Autodesk Inventor part; units mm, degrees
ref_plane "YZ Plane" through (0, 0, 0) normal (1, 0, 0) x (0, 1, 0)
ref_plane "XZ Plane" through (0, 0, 0) normal (0, 1, 0) x (-1, 0, 0)
ref_plane "XY Plane" through (0, 0, 0) normal (0, 0, 1) x (1, 0, 0)
sketch "Sketch1" plane through (0, 0, 0) normal (0, 0, 1) x (1, 0, 0)
  arc A0 (58.1571, 20) -> (-58.1571, 20) centre (0, 0) ccw
  line L0 (-90, 0) -> (90, 0) construction
  line L1 (-90, 20) -> (90, 20)
  line L2 (-90, 23) -> (90, 23)
  line L3 (-90, 20) -> (-90, 23)
  line L4 (90, 20) -> (90, 23)
  arc A1 (61.3209, 20) -> (-61.3209, 20) centre (0, 0) ccw
  point P0 (60.2599, 23)
  point P1 (-60.2599, 23)
  dimension "d8" = 123
  dimension "d12" = 90
  dimension "d13" = 90
  dimension "d14" = 0
  dimension "d15" = 20
  dimension "d16" = 3
  dimension "d17" = 129
  dimension "d18" = 180
  dimension "d19" = 90
extrude "Extrusion2" add sketch "Sketch1" against normal blind 20 contours A0 L2 A1 L1 | A0 L2 A1 | L1 A1 L2 A0 | A1 L2 L4 L1 | L1 L3 L2 A1
sketch "Sketch2" plane through (60.2599, 23, 0) normal (0, 1, 0) x (1, 0, 0)
  circle A0 centre (14, 10) radius 5
  line L0 (29.7401, 0) -> (0, 0)
  point P0 (-60.2599, 0)
  dimension "d22" = 10
  dimension "d23" = 10
  dimension "d24" = 14
hole "Hole1" at (74.2599, 23, -10) direction (0, -1, 0) diameter 10 end through all
ref_plane "Work Plane1" through (0, 20, 0) normal (1, 0, 0) x (0, 0, -1)
thread "Thread1"
mirror "Mirror1" about plane through (0, 20, 0) normal (1, 0, 0) of "Hole1"
properties part number "Holder"
Read the model definition and answer for the solid it produces. Units are mm, in the model's axes. A direction names the side the tool comes from. Coordinates: 2 decimals unless noted, no trailing zeros. Write each loop counter-clockwise with the first axis right and the second up, starting at its lowest first coordinate (ties: lowest second). Pieces come first, ordered by that corner, then holes. Notation, with made-up numbers: M 23,83.25 L 46,83.25 A30 ccw 46,106.25 Z; hole C 16,-0.5 d11. An arc over 180 degrees is marked long. Use a Markdown table: item, result.
Q1. The part is cut by section A-A, the plane z = -10. Write down the section's boundary in (x, y), then the cut area to 3 significant figures.
Answer block:
| item | result |
|---|---|
| outline | M -90,20 L -79.26,20 L -79.26,23 L -90,23 Z; M -69.26,20 L -58.16,20 A61.5 cw 58.16,20 L 69.26,20 L 69.26,23 L 60.26,23 A64.5 ccw -60.26,23 L -69.26,23 Z; M 79.26,20 L 90,20 L 90,23 L 79.26,23 Z |
| area | 587 mm2 |
Q2. Determine the mould class of faces 4 (the face through (0, 62, 0)), 5 (the face through (1.07, 61.49, -9.86)), 6 (the face through (-90, 21, -10)) for opening direction X: released by +X, released by -X, zero draft, split by the parting line, or undercut.
Answer block:
| item | result |
|---|---|
| face 4 | zero draft |
| face 5 | undercut |
| face 6 | released by -X |
Q3. The part is cut by section B-B, the plane y = 33. Write down the section's boundary in (x, z), then the cut area to 3 significant figures.
Answer block:
| item | result |
|---|---|
| outline | M -55.42,-20 L -51.9,-20 L -51.9,0 L -55.42,0 Z; M 51.9,-20 L 55.42,-20 L 55.42,0 L 51.9,0 Z |
| area | 141 mm2 |
Q4. The part is cut by section C-C, the plane y = 48. Write down the section's boundary in (x, z), then the cut area to 3 significant figures.
Answer block:
| item | result |
|---|---|
| outline | M -43.08,-20 L -38.45,-20 L -38.45,0 L -43.08,0 Z; M 38.45,-20 L 43.08,-20 L 43.08,0 L 38.45,0 Z |
| area | 185 mm2 |
Q5. Straight lines are drawn through the part: L1, parallel to X at y = 21.9, z = -10; L2, parallel to X at y = 22.3, z = -10; L3, parallel to X at y = 54, z = -11.5. For each, find the intervals that lie inside material, in ascending order. Write a range as [from, to].
Answer block:
| item | result |
|---|---|
| L1 | x = [-90, -79.26], [-69.26, -57.47], [57.47, 69.26], [79.26, 90] |
| L2 | x = [-90, -79.26], [-69.26, -57.31], [57.31, 69.26], [79.26, 90] |
| L3 | x = [-35.27, -29.43], [29.43, 35.27] |
Q6. The part is cut by section D-D, the plane x = 49.5. Write down the section's boundary in (y, z).
Answer block:
| item | result |
|---|---|
| outline | M 36.5,-20 L 41.35,-20 L 41.35,0 L 36.5,0 Z |
Q7. Each of these flat-tipped pins is pushed along its axis until it touches: pin 1 Ø10 at (x, z) = (3.5, -4.5) entering from -Y; pin 2 Ø1 at (x, z) = (-53, -12) entering from -Y; pin 3 Ø10 at (x, z) = (-71.5, -11.5) entering from +Y. Where does it stop, or does it pass through?
Answer block:
| item | result |
|---|---|
| pin 1 | stops at y = 60.91 |
| pin 2 | stops at y = 30.33 |
| pin 3 | stops at y = 23 |
Q8. Which of the six approach directions +Z, -Z, +X, -X, +Y, -Y give full straight-line access (tool end or side, diameter ignored) to faces 1 (the face through (72, 23, -5)), 2 (the face through (1.09, 64.49, -9.86)), 3 (the face through (-79, 23, -5))?
Answer block:
| item | result |
|---|---|
| face 1 | +Z, -Z, +X, +Y |
| face 2 | +Z, -Z, +Y |
| face 3 | +Z, -Z, -X, +Y |
